from build123d import *

# Parameters (mm, degrees)
SKETCH1_W           = 36
SKETCH1_H           = 29.7
SKETCH1_W_2         = 26.4
SKETCH1_H_2         = 6.9
BOSS_EXTRUDE1_DEPTH = 6.2
FILLET1_R           = 4
FILLET2_R           = 0.5


with BuildPart() as part:
    # Sketch1 → Boss-Extrude1 (new body)
    with BuildSketch(Plane(origin=(0, 0, 0), x_dir=(1, 0, 0), z_dir=(0, 1, 0))):
        with Locations((0, 8.6)):
            Rectangle(SKETCH1_W, SKETCH1_H)
        Rectangle(SKETCH1_W_2, SKETCH1_H_2, mode=Mode.SUBTRACT)
    extrude(amount=BOSS_EXTRUDE1_DEPTH)

    # Fillet1
    fillet1_edges = [part.edges().sort_by_distance(p)[0] for p in [
        (-18, 3.1, -23.45),
        (18, 3.1, -23.45),
        (18, 3.1, 6.25),
        (-18, 3.1, 6.25),
    ]]
    fillet(fillet1_edges, radius=FILLET1_R)

    # Fillet2
    fillet2_edges = [part.edges().sort_by_distance(p)[0] for p in [
        (13.2, 3.1, 3.45),
        (13.2, 3.1, -3.45),
        (-13.2, 3.1, -3.45),
        (-13.2, 3.1, 3.45),
    ]]
    fillet(fillet2_edges, radius=FILLET2_R)


solid = part.part
Geometry check sheet. Reference: the model listing, model coordinates, mm. A direction names the side the tool comes from. Round coordinates to 2 decimals unless told otherwise and drop trailing zeros. Write each loop counter-clockwise with the first axis right and the second up, starting at its lowest first coordinate (ties: lowest second). Pieces come first, ordered by that corner, then holes. Notation, with made-up numbers: (-33, 7) - (20, 7) arc R20 cw to (20, 31) - close; hole circle Ø9 at (40, 74.5). An arc over 180 degrees is marked (long way). One line per item, written item: value.
1. Cross-section at B-B on z = 1.5. Record the boundary of the cut face in (x, y), and give its area (3 significant figures).
The answers:
outline: (-18, 0) - (-13.2, 0) - (-13.2, 6.2) - (-18, 6.2) - close; (13.2, 0) - (18, 0) - (18, 6.2) - (13.2, 6.2) - close
area: 59.5 mm^2
2. Set-up check for faces 4 (the face through (0, 3, -23.45)), 5 (the face through (0, 3, -3.45)): record each of +Z, -Z, +X, -X, +Y, -Y from which the full face is reachable in a straight line by a thin tool's end or side.
The answers:
face 4: -Z, +X, -X, +Y, -Y
face 5: +Y, -Y
3. Cross-section at A-A on x = 1. Record the boundary of the cut face in (y, z), and give its area (3 significant figures).
The answers:
outline: (0, -23.45) - (6.2, -23.45) - (6.2, -3.45) - (0, -3.45) - close; (0, 3.45) - (6.2, 3.45) - (6.2, 6.25) - (0, 6.25) - close
area: 141 mm^2
4. Mould release check, pull along X, two halves, no side actions. Record for faces 1 (the face through (0, 0, -12)), 2 (the face through (0, 3, 3.45)), 3 (the face through (-16.859, 3.143, -22.247)): released by +X, released by -X, zero draft, split by the parting line, or undercut.
The answers:
face 1: zero draft
face 2: undercut
face 3: released by -X
5. Cross-section at C-C on y = 4. Record the boundary of the cut face in (x, z), and give its area (3 significant figures).
The answers:
outline: (-18, -19.45) arc R4 ccw to (-14, -23.45) - (14, -23.45) arc R4 ccw to (18, -19.45) - (18, 2.25) arc R4 ccw to (14, 6.25) - (-14, 6.25) arc R4 ccw to (-18, 2.25) - close; hole (-13.2, -2.95) arc R0.5 ccw to (-12.7, -3.45) - (12.7, -3.45) arc R0.5 ccw to (13.2, -2.95) - (13.2, 2.95) arc R0.5 ccw to (12.7, 3.45) - (-12.7, 3.45) arc R0.5 ccw to (-13.2, 2.95) - close
area: 874 mm^2
6. Depth check by flat-ended pin: pin 1 Ø2 at (x, z) = (11.5, -2) entering from -Y. Enter the tip coordinate at first touch or a pass-through.
The answers:
pin 1: passes through
7. Scan lines: L1, parallel to X at y = 2.5, z = 1; L2, parallel to Z at x = -11.5, y = 1; L3, parallel to Z at x = 15.5, y = 5.5. Record each from-to range of solid material in increasing order.
The answers:
L1: x = -18 to -13.2, 13.2 to 18
L2: z = -23.45 to -3.45, 3.45 to 6.25
L3: z = -23.16 to 5.96
